Build history of the part. All positions in model axes, mm. A direction names the side the tool comes from. Coordinates: 2 decimals unless noted, no trailing zeros. Order: outer loops, then holes, each group sorted by start corner. A loop starts at its lowest first (then second) coordinate and runs counter-clockwise, first axis right, second up. Notation, with made-up numbers: (57.25, 82) - (112.25, 82) arc R23 ccw to (112.25, 113) - close; hole circle Ø4 at (76, 39.5). An arc over 180 degrees is marked (long way). Return JSON: item names as keys, results as strings.
from build123d import *

# Parameters (mm, degrees)
BOSS_EXTRUDE1_DEPTH = 7.62
CIRPATTERN1_COUNT   = 16
SKETCH2_R           = 1.905
CUT_EXTRUDE1_DEPTH  = 8.6200001
SKETCH4_R           = 3.175
CUT_EXTRUDE2_DEPTH  = 3.81


with BuildPart() as part:
    # Sketch1 → Boss-Extrude1 (new body)
    with BuildSketch(Plane(origin=(0, 0, 0), x_dir=(1, 0, 0), z_dir=(0, 1, 0))):
        with BuildLine():
            add(Edge.make_bspline(
                [(1.139719329, 10.734666499), (1.147399116, 11.22537279), (0.871214241, 12.119041795), (0.344554873, 12.955131401), (0.094484742, 13.334665261)],
                knots=[0.007821969, 0.007821969, 0.007821969, 0.007821969, 0.5, 0.928051836, 0.928051836, 0.928051836, 0.928051836], degree=3))
            ThreePointArc((0.094484742, 13.334665261), (0, 13.335), (-0.094484742, 13.334665261))
            add(Edge.make_bspline(
                [(-1.139719329, 10.734666499), (-1.147399116, 11.22537279), (-0.871214241, 12.119041795), (-0.344554873, 12.955131401), (-0.094484742, 13.334665261)],
                knots=[0.007821969, 0.007821969, 0.007821969, 0.007821969, 0.5, 0.928051836, 0.928051836, 0.928051836, 0.928051836], degree=3))
            ThreePointArc((-1.139719329, 10.734666499), (0, -10.795), (1.139719329, 10.734666499))
        make_face()
    boss_extrude1 = extrude(amount=BOSS_EXTRUDE1_DEPTH)

    # CirPattern1: Boss-Extrude1 ×16 about axis
    cirpattern1_axis = Axis((0, 7.62, 0), (0, 1, 0))
    for i in range(1, CIRPATTERN1_COUNT):
        add(boss_extrude1.rotate(cirpattern1_axis, i * 360 / CIRPATTERN1_COUNT))

    # Sketch2 → Cut-Extrude1 (cut, through all)
    with BuildSketch(Plane(origin=(0, 7.62, 0), x_dir=(1, 0, 0), z_dir=(0, 1, 0))):
        Circle(SKETCH2_R)
    extrude(amount=-CUT_EXTRUDE1_DEPTH, mode=Mode.SUBTRACT)

    # Sketch4 → Cut-Extrude2 (cut)
    with BuildSketch(Plane.XZ):
        Circle(SKETCH4_R)
    extrude(amount=-CUT_EXTRUDE2_DEPTH, mode=Mode.SUBTRACT)


solid = part.part
1. Probe L1, parallel to X at y = 5, z = 0 (3 decimals); L2, parallel to Z at x = 0, y = 1.45 (3 decimals). List the from-to ranges inside material, lowest first.
Check values:
{"L1": "-13.335 to -1.905, 1.905 to 13.335", "L2": "-13.335 to -3.175, 3.175 to 13.335"}
2. Tool access for faces 4 (the cylindrical face through (-2.119, 3.757, 10.585)), 5 (the cylindrical face through (-2.09, 3.76, -10.59)), 6 (the cylindrical face through (-10.585, 3.757, -2.119)), 7 (the cylindrical face through (10.585, 3.757, 2.119)), 8 (the cylindrical face through (-0.69, 1.88, -3.1)): list every direction of +Z, -Z, +X, -X, +Y, -Y with a clear straight run to the whole face (end or side of a thin tool).
Check values:
{"face 4": "+Z, +Y, -Y", "face 5": "-Z, +Y, -Y", "face 6": "-X, +Y, -Y", "face 7": "+X, +Y, -Y", "face 8": "-Y"}
3. Drop flat-ended pins along their axis: pin 1 (5 mm diameter, centred on x = 0, z = 0, fed in from -Y); pin 2 (1 mm diameter, centred on y = 6.5, z = -9.5, fed in from -X); pin 3 (2 mm diameter, centred on x = 2.5, y = 5, fed in from -Z). Give the stop position or say it passes through.
Check values:
{"pin 1": "y = 3.81", "pin 2": "x = -9.5", "pin 3": "z = -11.09"}
4. Cut at A-A on x = -6. Give the cut face in (y, z).
Check values:
{"outline": "(0, -8.97) - (7.62, -8.97) - (7.62, 8.97) - (0, 8.97) - close"}
5. Mould opens along Z. For faces 1 (the cylindrical face through (2.119, 3.757, -10.585)), 2 (the cylindrical face through (-10.59, 3.76, 2.09)), 3 (the flat face through (2, 0, 4)) say: pulls with the +Z half, pulls with the -Z half, needs draft (parallel to the pull), parting line crosses it, or undercut.
Check values:
{"face 1": "pulls with the -Z half", "face 2": "undercut", "face 3": "needs draft"}
